```python
from build123d import *

# Parameters (mm, degrees)
SKETCH5_R           = 1.55
BOSS_EXTRUDE2_DEPTH = 1
BOSS_EXTRUDE3_START = -3
SKETCH6_R           = 1.55
BOSS_EXTRUDE3_DEPTH = 6
SKETCH11_R          = 3.05
SKETCH11_R_2        = 1.55
BOSS_EXTRUDE4_DEPTH = 3
CUT_EXTRUDE1_START  = 2
CUT_EXTRUDE1_DEPTH  = 6
SKETCH8_W           = 11
SKETCH8_H           = 8
SKETCH8_W_2         = 20
SKETCH8_H_2         = 12
CUT_EXTRUDE2_DEPTH  = 2
SKETCH9_W           = 0.45
SKETCH9_H           = 30
CUT_EXTRUDE3_DEPTH  = 3.5
CUT_EXTRUDE4_REACH  = 105.7
SKETCH10_W          = 30
SKETCH10_H          = 5.1


with BuildPart() as part:
    # Sweep1: sweep along a path in Sketch1
    with BuildLine(Plane(origin=(0, 0, 0), x_dir=(1, 0, 0), z_dir=(0, 1, 0))) as sweep1_path:
        Line((-48.26, -50.8), (48.26, -50.8))
        ThreePointArc((48.26, -50.8), (50.056051224, -50.056051224), (50.8, -48.26))
        Line((50.8, -48.26), (50.8, 48.26))
        ThreePointArc((50.8, 48.26), (50.056051224, 50.056051224), (48.26, 50.8))
        Line((48.26, 50.8), (-48.26, 50.8))
        ThreePointArc((-48.26, 50.8), (-50.056051224, 50.056051224), (-50.8, 48.26))
        Line((-50.8, 48.26), (-50.8, -48.26))
        ThreePointArc((-50.8, -48.26), (-50.056051224, -50.056051224), (-48.26, -50.8))
    # Sketch3 → Sweep1 (sweep)
    with BuildSketch(Plane.XY):
        Polygon((-50.85, 1.6), (-51.85, 1.6), (-51.85, -10), (-50.35, -10), (-50.35, 0), (-50.85, 0), align=None)
    sweep(path=sweep1_path.line)

    # Sketch5 → Boss-Extrude2 (add)
    with BuildSketch(Plane.XZ.offset(10)):
        with BuildLine():
            Line((-50.8, 48.26), (-50.8, -48.26))
            ThreePointArc((-50.8, -48.26), (-50.056051224, -50.056051224), (-48.26, -50.8))
            Line((-48.26, -50.8), (48.26, -50.8))
            ThreePointArc((48.26, -50.8), (50.056051224, -50.056051224), (50.8, -48.26))
            Line((50.8, -48.26), (50.8, 48.26))
            ThreePointArc((50.8, 48.26), (50.056051224, 50.056051224), (48.26, 50.8))
            Line((48.26, 50.8), (-48.26, 50.8))
            ThreePointArc((-48.26, 50.8), (-50.056051224, 50.056051224), (-50.8, 48.26))
        make_face()
        with Locations((-15.24, -24.384)):
            Circle(SKETCH5_R, mode=Mode.SUBTRACT)
        with Locations((29.972, 7.62)):
            Circle(SKETCH5_R, mode=Mode.SUBTRACT)
        with Locations((-20.4724, 24.13)):
            Circle(SKETCH5_R, mode=Mode.SUBTRACT)
    extrude(amount=-BOSS_EXTRUDE2_DEPTH)

    # Sketch6 → Boss-Extrude3 (add)
    with BuildSketch(Plane(origin=(0, 0, 0), x_dir=(1, 0, 0), z_dir=(0, 1, 0)).offset(BOSS_EXTRUDE3_START)):
        Polygon((-10.043847577, 24.384), (-12.641923789, 28.884), (-17.838076211, 28.884), (-20.436152423, 24.384), (-17.838076211, 19.884), (-12.641923789, 19.884), align=None)
        with Locations((-15.24, 24.384)):
            Circle(SKETCH6_R, mode=Mode.SUBTRACT)
        Polygon((35.168152423, -7.62), (32.570076211, -3.12), (27.373923789, -3.12), (24.775847577, -7.62), (27.373923789, -12.12), (32.570076211, -12.12), align=None)
        with Locations((29.972, -7.62)):
            Circle(SKETCH6_R, mode=Mode.SUBTRACT)
        Polygon((-15.276247577, -24.13), (-17.874323789, -19.63), (-23.070476211, -19.63), (-25.668552423, -24.13), (-23.070476211, -28.63), (-17.874323789, -28.63), align=None)
        with Locations((-20.4724, -24.13)):
            Circle(SKETCH6_R, mode=Mode.SUBTRACT)
    extrude(amount=-BOSS_EXTRUDE3_DEPTH)

    # Sketch11 → Boss-Extrude4 (add)
    with BuildSketch(Plane(origin=(0, -3, 0), x_dir=(1, 0, 0), z_dir=(0, 1, 0))):
        with Locations((-15.24, 24.384)):
            Circle(SKETCH11_R)
        with Locations((-15.24, 24.384)):
            Circle(SKETCH11_R_2, mode=Mode.SUBTRACT)
        with Locations((-20.4724, -24.13)):
            Circle(SKETCH11_R)
        with Locations((-20.4724, -24.13)):
            Circle(SKETCH11_R_2, mode=Mode.SUBTRACT)
        with Locations((29.972, -7.62)):
            Circle(SKETCH11_R)
        with Locations((29.972, -7.62)):
            Circle(SKETCH11_R_2, mode=Mode.SUBTRACT)
    extrude(amount=BOSS_EXTRUDE4_DEPTH)

    # Sketch7 → Cut-Extrude1 (cut, through all)
    with BuildSketch(Plane.XZ.offset(3).offset(CUT_EXTRUDE1_START)):
        Polygon((-17.239238493, 24.13), (-18.855819246, 26.93), (-22.088980754, 26.93), (-23.705561507, 24.13), (-22.088980754, 21.33), (-18.855819246, 21.33), align=None)
        Polygon((33.205161507, 7.62), (31.588580754, 10.42), (28.355419246, 10.42), (26.738838493, 7.62), (28.355419246, 4.82), (31.588580754, 4.82), align=None)
        Polygon((-12.006838493, -24.384), (-13.623419246, -21.584), (-16.856580754, -21.584), (-18.473161507, -24.384), (-16.856580754, -27.184), (-13.623419246, -27.184), align=None)
    extrude(amount=CUT_EXTRUDE1_DEPTH, mode=Mode.SUBTRACT)

    # Sketch8 → Cut-Extrude2 (cut, through all)
    with BuildSketch(Plane(origin=(0, -9, 0), x_dir=(1, 0, 0), z_dir=(0, 1, 0))):
        with Locations((-6.4408, 46.35)):
            Rectangle(SKETCH8_W, SKETCH8_H)
        with BuildLine():
            Line((50.35, -41.35), (50.35, -48.26))
            ThreePointArc((50.35, -48.26), (49.737853173, -49.737853173), (48.26, -50.35))
            Line((48.26, -50.35), (25.8, -50.35))
            Line((25.8, -50.35), (25.8, -41.35))
            Line((25.8, -41.35), (50.35, -41.35))
        make_face()
        with Locations((27.35, 44.35)):
            Rectangle(SKETCH8_W_2, SKETCH8_H_2)
    extrude(amount=-CUT_EXTRUDE2_DEPTH, mode=Mode.SUBTRACT)

    # Sketch9 → Cut-Extrude3 (cut)
    with BuildSketch(Plane(origin=(0, 0, 0), x_dir=(1, 0, 0), z_dir=(0, 1, 0))):
        with Locations((50.575, -26.8)):
            Rectangle(SKETCH9_W, SKETCH9_H)
    extrude(amount=-CUT_EXTRUDE3_DEPTH, mode=Mode.SUBTRACT)

    # Sketch10 → Cut-Extrude4 (cut, up to next)
    with BuildSketch(Plane(origin=(51.85, 0, 0), x_dir=(0, 0, -1), z_dir=(1, 0, 0)), mode=Mode.PRIVATE) as cut_extrude4_sk1:
        with Locations((-26.8, -0.95)):
            Rectangle(SKETCH10_W, SKETCH10_H)
    cut_extrude4_tool1 = extrude(cut_extrude4_sk1.sketch, amount=-CUT_EXTRUDE4_REACH, mode=Mode.PRIVATE) & part.part
    add(cut_extrude4_tool1.solids().sort_by_distance((51.85, -0.95, 26.8))[0], mode=Mode.SUBTRACT)


solid = part.part
```
Geometry check sheet. Reference: the model listing, model coordinates, mm. A direction names the side the tool comes from. Give positions to 0.01 mm unless a question says otherwise; leave off trailing zeros. Write each loop counter-clockwise with the first axis right and the second up, starting at its lowest first coordinate (ties: lowest second). Pieces come first, ordered by that corner, then holes.
1) Material ranges on L1, parallel to X at y = -3.1, z = 7.62; L2, parallel to X at y = -2.75, z = -46, recorded low to high.
2) Section check A-A, the plane x = -6. Record the boundary of the cut face in (y, z), and give its area (3 significant figures).
3) Section check D-D, the plane x = -28. Record the boundary of the cut face in (y, z).
4) Section check B-B, the plane y = -6.5. State how many separate pieces and enclosed holes the cut face has, and give its area (3 significant figures).
5) Section check C-C, the plane z = -34.5. Record the boundary of the cut face in (x, y), and give its area (3 significant figures).
6) Gauge pin test, flat ends, axial feed: pin 1 (1.2 mm diameter, centred on x = 51, y = -2, fed in from -Z); pin 2 (4.5 mm diameter, centred on x = -21.5, z = 23, fed in from -Y); pin 3 (4.5 mm diameter, centred on x = -19.5, z = 23, fed in from +Y); pin 4 (5 mm diameter, centred on x = -20.47, z = 24.13, fed in from -Y). Record the tip position at first contact, or that the pin passes through.
7) Release check for a two-part mould opening along X. For faces 1 (the cylindrical face through (28.74, -2.54, 8.56)), 2 (the flat face through (1, -10, 1)), 3 (the cylindrical face through (-50.826, -4.281, 50.77)), 4 (the flat face through (31.1, -3, 4.6)) record: pulls with the +X half, pulls with the -X half, needs draft (parallel to the pull), parting line crosses it, or undercut.
8) Access from +Z, -Z, +X, -X, +Y, -Y to the whole of each face (thin tool, end or side, straight path). Record for faces 5 (the flat face through (-11.361, -5.958, -22.102)), 6 (the flat face through (-22, 0, 23)), 7 (the flat face through (27.536, -7.465, 6.24)).
Computed:
1. L1: x = -51.85 to -50.35, 24.78 to 28.42, 31.52 to 35.17, 50.35 to 51.85
1. L2: x = -51.85 to -50.35, 50.35 to 51.85
2. outline: (-10, -51.85) - (1.6, -51.85) - (1.6, -50.85) - (0, -50.85) - (0, -50.35) - (-10, -50.35) - close; (-10, -42.35) - (-9, -42.35) - (-9, 50.35) - (0, 50.35) - (0, 50.85) - (1.6, 50.85) - (1.6, 51.85) - (-10, 51.85) - close
2. area: 126 mm2
3. outline: (-10, -51.85) - (1.6, -51.85) - (1.6, -50.85) - (0, -50.85) - (0, -50.35) - (-9, -50.35) - (-9, 50.35) - (0, 50.35) - (0, 50.85) - (1.6, 50.85) - (1.6, 51.85) - (-10, 51.85) - close
4. separate pieces: 4
4. enclosed holes: 4
4. area: 735 mm2
5. outline: (-51.85, -10) - (51.85, -10) - (51.85, 1.6) - (50.85, 1.6) - (50.85, 0) - (50.35, 0) - (50.35, -9) - (-50.35, -9) - (-50.35, 0) - (-50.85, 0) - (-50.85, 1.6) - (-51.85, 1.6) - close
5. area: 134 mm2
6. pin 1: stops at z = -51.14
6. pin 2: stops at y = -10
6. pin 3: stops at y = 0
6. pin 4: stops at y = -5
7. face 1: undercut
7. face 2: needs draft
7. face 3: pulls with the -X half
7. face 4: undercut
8. face 5: +Y
8. face 6: +X, +Y
8. face 7: -Y
